```python
from build123d import *

# Parameters (mm, degrees)
SALIENTE_EXTRUIR1_DEPTH = 4
CROQUIS2_R              = 1.5
CORTAR_EXTRUIR1_DEPTH   = 10
CROQUIS3_R              = 1.5
CROQUIS3_R_2            = 1.439143575
CORTAR_EXTRUIR2_DEPTH   = 10
CROQUIS4_R              = 1.620915762
CROQUIS4_R_2            = 1.5
CORTAR_EXTRUIR3_DEPTH   = 50
CROQUIS5_R              = 5
CORTAR_EXTRUIR4_DEPTH   = 10


with BuildPart() as part:
    # Croquis1 → Saliente-Extruir1 (new body)
    with BuildSketch(Plane(origin=(0, 0, 0), x_dir=(1, 0, 0), z_dir=(0, 1, 0))):
        Polygon((-90, 81), (-124.5, 47), (-124.5, -47), (-90, -81), (0, -81), (90, -81), (124.5, -47), (124.5, 47), (90, 81), (0, 81), align=None)
    extrude(amount=SALIENTE_EXTRUIR1_DEPTH)

    # Croquis2 → Cortar-Extruir1 (cut)
    with BuildSketch(Plane(origin=(0, 4, 0), x_dir=(1, 0, 0), z_dir=(0, 1, 0))):
        with Locations(Location((-85, 63.060809699, 0), (0, 0, 270))):
            Circle(CROQUIS2_R)
        with Locations(Location((-85, -63.060809699, 0), (0, 0, 270))):
            Circle(CROQUIS2_R)
        with Locations(Location((85, -63.060809699, 0), (0, 0, 270))):
            Circle(CROQUIS2_R)
        with Locations(Location((85, 63.060809699, 0), (0, 0, 270))):
            Circle(CROQUIS2_R)
    extrude(amount=-CORTAR_EXTRUIR1_DEPTH, mode=Mode.SUBTRACT)

    # Croquis3 → Cortar-Extruir2 (cut)
    with BuildSketch(Plane(origin=(0, 4, 0), x_dir=(1, 0, 0), z_dir=(0, 1, 0))):
        with Locations(Location((94.732844127, -62.29571743, 0), (0, 0, 270))):
            Circle(CROQUIS3_R)
        with Locations(Location((77.563491473, -44.873874295, 0), (0, 0, 270))):
            Circle(CROQUIS3_R)
        with Locations(Location((77.563491473, 44.873874295, 0), (0, 0, 270))):
            Circle(CROQUIS3_R_2)
        with Locations(Location((94.732844127, 62.29571743, 0), (0, 0, 270))):
            Circle(CROQUIS3_R)
    extrude(amount=-CORTAR_EXTRUIR2_DEPTH, mode=Mode.SUBTRACT)

    # Croquis4 → Cortar-Extruir3 (cut)
    with BuildSketch(Plane.XZ):
        with Locations(Location((-65.16861846, -77.381821896, 0), (0, 0, 270))):
            Circle(CROQUIS4_R)
        with Locations(Location((-51.026482836, -63.239686272, 0), (0, 0, 270))):
            Circle(CROQUIS4_R_2)
        with Locations(Location((-65.16861846, 77.381821896, 0), (0, 0, 270))):
            Circle(CROQUIS4_R_2)
        with Locations(Location((-51.026482836, 63.239686272, 0), (0, 0, 270))):
            Circle(CROQUIS4_R_2)
    extrude(amount=-CORTAR_EXTRUIR3_DEPTH, mode=Mode.SUBTRACT)

    # Croquis5 → Cortar-Extruir4 (cut)
    with BuildSketch(Plane(origin=(0, 4, 0), x_dir=(1, 0, 0), z_dir=(0, 1, 0))):
        with Locations(Location((0, 0, 0), (0, 0, 270))):
            Circle(CROQUIS5_R)
    extrude(amount=-CORTAR_EXTRUIR4_DEPTH, mode=Mode.SUBTRACT)


solid = part.part
```
Check sheet for the modelled part. Datum: model origin and axes. Units: mm. Coordinates: 2 decimals unless noted, no trailing zeros. Write each loop counter-clockwise with the first axis right and the second up, starting at its lowest first coordinate (ties: lowest second). Pieces come first, ordered by that corner, then holes. Notation, with made-up numbers: (-7, 5) -> (25, 5) arc R13 ccw to (25, 19) -> close; hole circle Ø3 at (58.25, 51.5). An arc over 180 degrees is marked (long way). Use a Markdown table: item, result.
1. Sectioned sample at A-A (x = 0). Enter the section's corners in (y, z), plus the area to 3 significant figures.
Reported:
| item | result |
|---|---|
| outline | (0, -81) -> (4, -81) -> (4, -5) -> (0, -5) -> close; (0, 5) -> (4, 5) -> (4, 81) -> (0, 81) -> close |
| area | 608 mm2 |
2. Sectioned sample at B-B (y = 2.1). Give the number of separate pieces and of enclosed holes in the cut face, plus the area to 3 significant figures.
Reported:
| item | result |
|---|---|
| separate pieces | 1 |
| enclosed holes | 13 |
| area | 37,800 mm2 |
3. Release check for a two-part mould opening along Z. For faces 1 (the flat face through (-107.008, 1.972, -64.238)), 2 (the flat face through (-107.492, 1.972, 63.762)), 3 (the cylindrical face through (-4.88, 2.03, -1.08)), 4 (the flat face through (-2, 4, -19)) record: pulls with the +Z half, pulls with the -Z half, needs draft (parallel to the pull), parting line crosses it, or undercut.
Reported:
| item | result |
|---|---|
| face 1 | pulls with the -Z half |
| face 2 | pulls with the +Z half |
| face 3 | undercut |
| face 4 | needs draft |
4. Sectioned sample at C-C (z = -58). Enter the section's corners in (x, y).
Reported:
| item | result |
|---|---|
| outline | (-113.34, 0) -> (113.34, 0) -> (113.34, 4) -> (-113.34, 4) -> close |
5. Go/stop test with flat-tipped pins: pin 1 Ø1 at (y, z) = (2, 49) entering from -X; pin 2 Ø1.5 at (y, z) = (3, 56) entering from +X. Record where each tip stops, or that it passes through.
Reported:
| item | result |
|---|---|
| pin 1 | stops at x = -122.98 |
| pin 2 | stops at x = 116.13 |
6. Scan lines: line 1 along Z through (x, y) = (85, 0.8); line 2 along Z through (x, y) = (78.5, 1.45); line 3 along X through (y, z) = (2.75, -49). Record each from-to range of solid material in increasing order.
Reported:
| item | result |
|---|---|
| line 1 | z = -81 to -64.56, -61.56 to 61.56, 64.56 to 81 |
| line 2 | z = -81 to -45.97, -43.78 to 43.7, 46.05 to 81 |
| line 3 | x = -122.47 to 122.47 |
